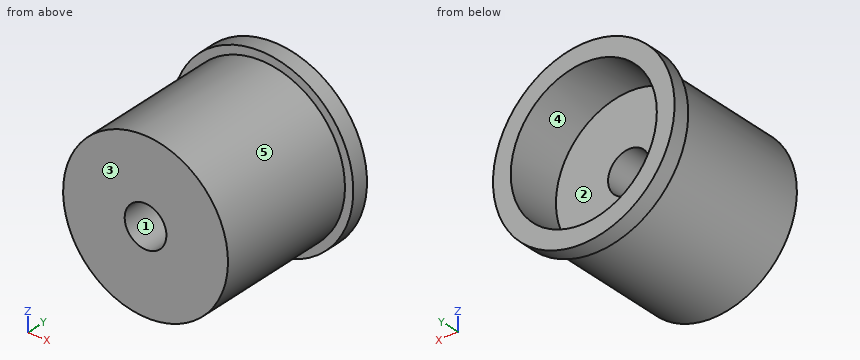
from build123d import *

# Parameters (mm, degrees)
SKETCH_1_R          = 19.75
EXTRUDE_1_DEPTH     = 34.2
SKETCH_2_R          = 21.75
EXTRUDE_2_DEPTH     = 4
SKETCH_3_R          = 5
CUT_EXTRUDE_1_DEPTH = 25
SKETCH_4_R          = 17.5
CUT_EXTRUDE_3_DEPTH = 13.2


with BuildPart() as part:
    # 草图1 → 凸台-拉伸1 (new body)
    with BuildSketch(Plane(origin=(0, 0, 0), x_dir=(1, 0, 0), z_dir=(0, 1, 0))):
        with Locations(Location((0, 0, 0), (0, 0, 270))):
            Circle(SKETCH_1_R)
    extrude(amount=EXTRUDE_1_DEPTH)

    # 草图2 → 凸台-拉伸2 (add)
    with BuildSketch(Plane(origin=(0, 34.2, 0), x_dir=(1, 0, 0), z_dir=(0, 1, 0))):
        with Locations(Location((0, 0, 0), (0, 0, 270))):
            Circle(SKETCH_2_R)
    extrude(amount=EXTRUDE_2_DEPTH)

    # 草图3 → 切除-拉伸1 (cut)
    with BuildSketch(Plane.XZ):
        with Locations(Location((0, 0, 0), (0, 0, 270))):
            Circle(SKETCH_3_R)
    extrude(amount=-CUT_EXTRUDE_1_DEPTH, mode=Mode.SUBTRACT)

    # 草图4 → 切除-拉伸3 (cut)
    with BuildSketch(Plane(origin=(0, 38.2, 0), x_dir=(1, 0, 0), z_dir=(0, 1, 0))):
        with Locations(Location((0, 0, 0), (0, 0, 270))):
            Circle(SKETCH_4_R)
    extrude(amount=-CUT_EXTRUDE_3_DEPTH, mode=Mode.SUBTRACT)


solid = part.part
Check sheet for the modelled part. Datum: model origin and axes. Units: mm. Face numbers are marked on the shaded views. A direction names the side the tool comes from. Coordinates: 2 decimals unless noted, no trailing zeros. Loops run counter-clockwise (first coordinate to the right, second up) from the corner with the lowest first, then second, coordinate; pieces in that order, holes last. Notation, with made-up numbers: (-15.75, 58) -> (40.25, 58) arc R20 ccw to (40.25, 78) -> close; hole circle Ø3 at (52, 42.25). An arc over 180 degrees is marked (long way). Write item = value, one per line. Start each with the question number.
1. Tool access check on the marked faces 1 and 2. Record the directions out of +Z, -Z, +X, -X, +Y, -Y that give a thin tool (end or side, any length) a straight path to the whole face; none if there is none.
2. Material ranges on line 1 (X direction, y = 7, z = 0); line 2 (X direction, y = 35, z = 0); line 3 (Y direction, x = -6, z = 6), recorded low to high.
3. Section check A-A on z = 0. Record the cut outline in (x, y).
4. Draft check along Z on the marked faces 3, 4 and 5. Enter one of: released by +Z, released by -Z, zero draft, split by the parting line, or undercut.
5. Section check C-C on y = 9. Record the cut outline in (x, z), then the cut area to 3 significant figures.
6. Depth check by flat-ended pin: P1, Ø1, axis at y = 19.5, z = -17.5, coming from the -X side; P2, Ø6, axis at y = 11.5, z = -1.5, coming from the +X side; P3, Ø16, axis at x = 0, z = 0, coming from the +Y side. Enter the tip coordinate at first touch or a pass-through.
7. Section check D-D on x = -10. Record the cut outline in (y, z), then the cut area to 3 significant figures.
8. Section check B-B on x = 0. Record the cut outline in (y, z).
Responses:
q1.face_1 = +Y, -Y
q1.face_2 = +Y
q2.line_1 = -19.75 to -5, 5 to 19.75
q2.line_2 = -21.75 to -17.5, 17.5 to 21.75
q2.line_3 = 0 to 25
q3.outline = (-21.75, 34.2) -> (-19.75, 34.2) -> (-19.75, 0) -> (-5, 0) -> (-5, 25) -> (-17.5, 25) -> (-17.5, 38.2) -> (-21.75, 38.2) -> close; (5, 0) -> (19.75, 0) -> (19.75, 34.2) -> (21.75, 34.2) -> (21.75, 38.2) -> (17.5, 38.2) -> (17.5, 25) -> (5, 25) -> close
q4.face_3 = zero draft
q4.face_4 = undercut
q4.face_5 = split by the parting line
q5.outline = circle Ø39.5 at (0, 0); hole circle Ø10 at (0, 0)
q5.area = 1,150 mm2
q6.P1 = -10.05
q6.P2 = 19.75
q6.P3 = 25
q7.outline = (0, -17.03) -> (34.2, -17.03) -> (34.2, -19.31) -> (38.2, -19.31) -> (38.2, -14.36) -> (25, -14.36) -> (25, 14.36) -> (38.2, 14.36) -> (38.2, 19.31) -> (34.2, 19.31) -> (34.2, 17.03) -> (0, 17.03) -> close
q7.area = 940 mm2
q8.outline = (0, -19.75) -> (34.2, -19.75) -> (34.2, -21.75) -> (38.2, -21.75) -> (38.2, -17.5) -> (25, -17.5) -> (25, -5) -> (0, -5) -> close; (0, 5) -> (25, 5) -> (25, 17.5) -> (38.2, 17.5) -> (38.2, 21.75) -> (34.2, 21.75) -> (34.2, 19.75) -> (0, 19.75) -> close
